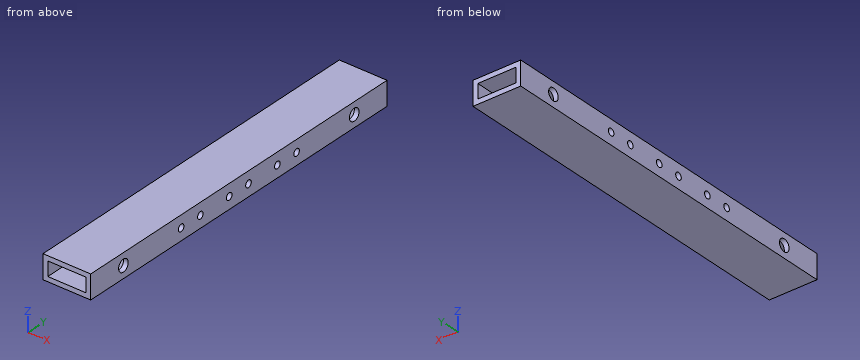
from build123d import *

# Parameters (mm, degrees)
SKETCH_1_W          = 20
SKETCH_1_H          = 10
SKETCH_1_W_2        = 16
SKETCH_1_H_2        = 6
EXTRUDE_1_DEPTH     = 77
SKETCH_2_R          = 1.45
SKETCH_2_R_2        = 2.5
CUT_EXTRUDE_1_DEPTH = 80.711981534


with BuildPart() as part:
    # 草图1 → 凸台-拉伸1 (new, symmetric)
    with BuildSketch(Plane(origin=(0, 0, 0), x_dir=(1, 0, 0), z_dir=(0, 1, 0))):
        Rectangle(SKETCH_1_W, SKETCH_1_H)
        Rectangle(SKETCH_1_W_2, SKETCH_1_H_2, mode=Mode.SUBTRACT)
    extrude(amount=EXTRUDE_1_DEPTH, both=True)

    # 草图2 → 切除-拉伸1 (cut, through all)
    with BuildSketch(Plane(origin=(10, 0, 0), x_dir=(0, 0, -1), z_dir=(1, 0, 0))):
        with Locations((0, 5)):
            Circle(SKETCH_2_R)
        with Locations((0, 20)):
            Circle(SKETCH_2_R)
        with Locations((0, 30)):
            Circle(SKETCH_2_R)
        with Locations((0, -30)):
            Circle(SKETCH_2_R)
        with Locations((0, -20)):
            Circle(SKETCH_2_R)
        with Locations((0, -5)):
            Circle(SKETCH_2_R)
        with Locations((0, 60)):
            Circle(SKETCH_2_R_2)
        with Locations((0, -60)):
            Circle(SKETCH_2_R_2)
    extrude(amount=-CUT_EXTRUDE_1_DEPTH, mode=Mode.SUBTRACT)


solid = part.part
The model under review builds one solid part; all positions refer to its coordinate system, in mm. Round coordinates to 2 decimals unless told otherwise and drop trailing zeros. Loops run counter-clockwise (first coordinate to the right, second up) from the corner with the lowest first, then second, coordinate; pieces in that order, holes last. Notation, with made-up numbers: (4.25, 57.25) -> (36.25, 57.25) arc R9 ccw to (36.25, 67.25) -> close; hole circle Ø9 at (59, 50.25). An arc over 180 degrees is marked (long way). One line per question, with ' | ' between items. Start each with the question number.
Item 1: Add section D-D, the plane y = -20. Write out the cut boundary in (x, z), then the cut area to 3 significant figures.
Item 2: Add section B-B, the plane x = -0.75. Write out the cut boundary in (y, z), then the cut area to 3 significant figures.
Item 3: Wall thickness on line 1 along Z through (x, y) = (7.25, 53.5); line 2 along X through (y, z) = (-49.5, 2); line 3 along Z through (x, y) = (-9, -31): over which ranges is each line inside the solid? List them lowest first. Write a range as [from, to].
Item 4: Add section A-A, the plane y = 60. Write out the cut boundary in (x, z), then the cut area to 3 significant figures.
Item 5: Add section C-C, the plane z = 0. Count the separate pieces of the cut face and the enclosed holes in it, then the cut area to 3 significant figures.
Return value:
1) outline: (-10, -5) -> (10, -5) -> (10, -1.45) -> (8, -1.45) -> (8, -3) -> (-8, -3) -> (-8, -1.45) -> (-10, -1.45) -> close; (-10, 1.45) -> (-8, 1.45) -> (-8, 3) -> (8, 3) -> (8, 1.45) -> (10, 1.45) -> (10, 5) -> (-10, 5) -> close | area: 92.4 mm2
2) outline: (-77, -5) -> (77, -5) -> (77, -3) -> (-77, -3) -> close; (-77, 3) -> (77, 3) -> (77, 5) -> (-77, 5) -> close | area: 616 mm2
3) line 1: z = [-5, -3], [3, 5] | line 2: x = [-10, -8], [8, 10] | line 3: z = [-5, -1.05], [1.05, 5]
4) outline: (-10, -5) -> (10, -5) -> (10, -2.5) -> (8, -2.5) -> (8, -3) -> (-8, -3) -> (-8, -2.5) -> (-10, -2.5) -> close; (-10, 2.5) -> (-8, 2.5) -> (-8, 3) -> (8, 3) -> (8, 2.5) -> (10, 2.5) -> (10, 5) -> (-10, 5) -> close | area: 84.0 mm2
5) separate pieces: 18 | enclosed holes: 0 | area: 506 mm2
